from build123d import *

# Parameters (mm, degrees)
SKETCH1_W                      = 80
SKETCH1_H                      = 100
BASE_FLANGE1_DEPTH             = 3.175
EDGE_FLANGE2_STRIP_W           = 14.1732
EDGE_FLANGE2_STRIP_H           = 3.175
EDGE_FLANGE2_STRIP_CUT_DEPTH   = 80
EDGE_FLANGE2_STRIP_2_W         = 14.1732
EDGE_FLANGE2_STRIP_2_H         = 3.175
EDGE_FLANGE2_STRIP_CUT_2_DEPTH = 80
EDGE_FLANGE2_DEPTH             = 80
EDGE_FLANGE2_BEND_DEPTH        = 80
CUT_EXTRUDE1_REACH             = 155.948
SKETCH12_R                     = 28
M6_CLEARANCE_HOLE1_D           = 6.4
M6_CLEARANCE_HOLE1_DEPTH       = 3.175
M6_CLEARANCE_HOLE2_D           = 6.4
CUT_EXTRUDE2_REACH             = 155.948
SKETCH19_R                     = 11
FILLET1_R                      = 5


# Sheet-metal steps are written as plain solids
with BuildPart() as part:
    # Sketch1 → Base-Flange1 (new body)
    with BuildSketch(Plane(origin=(0, 0, 0), x_dir=(0, 0, -1), z_dir=(0, -1, 0))):
        Rectangle(SKETCH1_W, SKETCH1_H)
    extrude(amount=-BASE_FLANGE1_DEPTH)

    # Edge-Flange2 strip (across the edge) → Edge-Flange2 strip cut (cut)
    with BuildSketch(Plane(origin=(50, 3.175, 40), x_dir=(-1, 0, 0), z_dir=(0, 0, -1))):
        with Locations((-3.175, -1.5875)):
            Rectangle(EDGE_FLANGE2_STRIP_W, EDGE_FLANGE2_STRIP_H)
    extrude(amount=EDGE_FLANGE2_STRIP_CUT_DEPTH, mode=Mode.SUBTRACT)

    # Edge-Flange2 strip 2 (across the edge) → Edge-Flange2 strip cut 2 (cut)
    with BuildSketch(Plane(origin=(-50, 3.175, -40), x_dir=(1, 0, 0), z_dir=(0, 0, 1))):
        with Locations((-3.175, -1.5875)):
            Rectangle(EDGE_FLANGE2_STRIP_2_W, EDGE_FLANGE2_STRIP_2_H)
    extrude(amount=EDGE_FLANGE2_STRIP_CUT_2_DEPTH, mode=Mode.SUBTRACT)

    # Edge-Flange2 section (across the edge) → Edge-Flange2 (add)
    with BuildSketch(Plane(origin=(50, 3.175, 40), x_dir=(-1, 0, 0), z_dir=(0, 0, -1))):
        with BuildLine():
            Line((0, 0.7366), (0, 106.825))
            Line((0, 106.825), (3.175, 106.825))
            Line((3.175, 106.825), (3.175, 0.7366))
            ThreePointArc((3.175, 0.7366), (3.390745145, 0.215745145), (3.9116, 0))
            Line((3.9116, 0), (3.9116, -3.175))
            ThreePointArc((3.9116, -3.175), (1.145681115, -2.029318885), (0, 0.7366))
        make_face()
    extrude(amount=EDGE_FLANGE2_DEPTH)

    # Edge-Flange2 section 2 (across the edge) → Edge-Flange2 bend (add)
    with BuildSketch(Plane(origin=(-50, 3.175, -40), x_dir=(1, 0, 0), z_dir=(0, 0, 1))):
        with BuildLine():
            Line((0, 0.7366), (0, 106.825))
            Line((0, 106.825), (3.175, 106.825))
            Line((3.175, 106.825), (3.175, 0.7366))
            ThreePointArc((3.175, 0.7366), (3.390745145, 0.215745145), (3.9116, 0))
            Line((3.9116, 0), (3.9116, -3.175))
            ThreePointArc((3.9116, -3.175), (1.145681115, -2.029318885), (0, 0.7366))
        make_face()
    extrude(amount=EDGE_FLANGE2_BEND_DEPTH)

    # Sketch12 → Cut-Extrude1 (cut, up to next)
    with BuildSketch(Plane(origin=(50, 0, 0), x_dir=(0, 0, -1), z_dir=(1, 0, 0)), mode=Mode.PRIVATE) as cut_extrude1_sk1:
        with BuildLine():
            Line((-40, 110), (-40, 70))
            ThreePointArc((-40, 70), (-28.284271269, 98.284271226), (-6.1e-08, 110))
            Line((-6.1e-08, 110), (-40, 110))
        make_face()
    cut_extrude1_tool1 = extrude(cut_extrude1_sk1.sketch, amount=-CUT_EXTRUDE1_REACH, mode=Mode.PRIVATE) & part.part
    # Sketch12 → Cut-Extrude1 (cut, up to next)
    with BuildSketch(Plane(origin=(50, 0, 0), x_dir=(0, 0, -1), z_dir=(1, 0, 0)), mode=Mode.PRIVATE) as cut_extrude1_sk2:
        with BuildLine():
            Line((40, 110), (-6.1e-08, 110))
            ThreePointArc((-6.1e-08, 110), (28.284271226, 98.284271269), (40, 70))
            Line((40, 70), (40, 110))
        make_face()
    cut_extrude1_tool2 = extrude(cut_extrude1_sk2.sketch, amount=-CUT_EXTRUDE1_REACH, mode=Mode.PRIVATE) & part.part
    # Sketch12 → Cut-Extrude1 (cut, up to next)
    with BuildSketch(Plane(origin=(50, 0, 0), x_dir=(0, 0, -1), z_dir=(1, 0, 0)), mode=Mode.PRIVATE) as cut_extrude1_sk3:
        with Locations(Location((0, 70, 0), (0, 0, 90))):
            Circle(SKETCH12_R)
    cut_extrude1_tool3 = extrude(cut_extrude1_sk3.sketch, amount=-CUT_EXTRUDE1_REACH, mode=Mode.PRIVATE) & part.part
    add(cut_extrude1_tool1.solids().sort_by_distance((50, 101.065282, 31.065282))[0], mode=Mode.SUBTRACT)
    add(cut_extrude1_tool2.solids().sort_by_distance((50, 101.065282, -31.065282))[0], mode=Mode.SUBTRACT)
    add(cut_extrude1_tool3.solids().sort_by_distance((50, 70, 0))[0], mode=Mode.SUBTRACT)

    # M6 Clearance Hole1
    with Locations(Plane(origin=(50, 70, 32.5), x_dir=(0, 1, 0), z_dir=(1, 0, 0))):
        with Locations((0, 0), (-32.5, -32.5), (0, -65), (32.5, -32.5)):
            Hole(M6_CLEARANCE_HOLE1_D / 2, depth=M6_CLEARANCE_HOLE1_DEPTH)

    # M6 Clearance Hole2 (through all)
    with Locations(Plane(origin=(-35, 0, 30), x_dir=(0, 0, -1), z_dir=(0, -1, 0))):
        with Locations((0, 0), (0, 70), (60, 0), (60, 70)):
            Hole(M6_CLEARANCE_HOLE2_D / 2)

    # Sketch19 → Cut-Extrude2 (cut, up to next)
    with BuildSketch(Plane.ZY.offset(50), mode=Mode.PRIVATE) as cut_extrude2_sk1:
        with BuildLine():
            Line((-40, 40), (-17.398181668, 79.864242224))
            ThreePointArc((-17.398181668, 79.864242224), (0, 90), (17.398181668, 79.864242224))
            Line((17.398181668, 79.864242224), (40, 40))
            Line((40, 40), (40, 110))
            Line((40, 110), (-40, 110))
            Line((-40, 110), (-40, 40))
        make_face()
    cut_extrude2_tool1 = extrude(cut_extrude2_sk1.sketch, amount=-CUT_EXTRUDE2_REACH, mode=Mode.PRIVATE) & part.part
    # Sketch19 → Cut-Extrude2 (cut, up to next)
    with BuildSketch(Plane.ZY.offset(50), mode=Mode.PRIVATE) as cut_extrude2_sk2:
        with Locations(Location((0, 70, 0), (0, 0, 270))):
            Circle(SKETCH19_R)
    cut_extrude2_tool2 = extrude(cut_extrude2_sk2.sketch, amount=-CUT_EXTRUDE2_REACH, mode=Mode.PRIVATE) & part.part
    # Sketch19 → Cut-Extrude2 (cut, up to next)
    with BuildSketch(Plane.ZY.offset(50), mode=Mode.PRIVATE) as cut_extrude2_sk3:
        with BuildLine():
            ThreePointArc((-11.390381057, 62), (-12.990381057, 60.4), (-14.590381057, 62))
            Line((-14.590381057, 62), (-14.590381057, 63))
            ThreePointArc((-14.590381057, 63), (-12.990381057, 64.6), (-11.390381057, 63))
            Line((-11.390381057, 63), (-11.390381057, 62))
        make_face()
    cut_extrude2_tool3 = extrude(cut_extrude2_sk3.sketch, amount=-CUT_EXTRUDE2_REACH, mode=Mode.PRIVATE) & part.part
    # Sketch19 → Cut-Extrude2 (cut, up to next)
    with BuildSketch(Plane.ZY.offset(50), mode=Mode.PRIVATE) as cut_extrude2_sk4:
        with BuildLine():
            ThreePointArc((14.590381057, 62), (12.990381057, 60.4), (11.390381057, 62))
            Line((11.390381057, 62), (11.390381057, 63))
            ThreePointArc((11.390381057, 63), (12.990381057, 64.6), (14.590381057, 63))
            Line((14.590381057, 63), (14.590381057, 62))
        make_face()
    cut_extrude2_tool4 = extrude(cut_extrude2_sk4.sketch, amount=-CUT_EXTRUDE2_REACH, mode=Mode.PRIVATE) & part.part
    # Sketch19 → Cut-Extrude2 (cut, up to next)
    with BuildSketch(Plane.ZY.offset(50), mode=Mode.PRIVATE) as cut_extrude2_sk5:
        with BuildLine():
            ThreePointArc((1.6, 84.5), (0, 82.9), (-1.6, 84.5))
            Line((-1.6, 84.5), (-1.6, 85.5))
            ThreePointArc((-1.6, 85.5), (0, 87.1), (1.6, 85.5))
            Line((1.6, 85.5), (1.6, 84.5))
        make_face()
    cut_extrude2_tool5 = extrude(cut_extrude2_sk5.sketch, amount=-CUT_EXTRUDE2_REACH, mode=Mode.PRIVATE) & part.part
    add(cut_extrude2_tool1.solids().sort_by_distance((-50, 60.456413, -29.623817))[0], mode=Mode.SUBTRACT)
    add(cut_extrude2_tool2.solids().sort_by_distance((-50, 70, 0))[0], mode=Mode.SUBTRACT)
    add(cut_extrude2_tool3.solids().sort_by_distance((-50, 62.5, -12.990381))[0], mode=Mode.SUBTRACT)
    add(cut_extrude2_tool4.solids().sort_by_distance((-50, 62.5, 12.990381))[0], mode=Mode.SUBTRACT)
    add(cut_extrude2_tool5.solids().sort_by_distance((-50, 85, 0))[0], mode=Mode.SUBTRACT)

    # Fillet1
    fillet1_edges = [part.edges().sort_by_distance(p)[0] for p in [
        (-48.4125, 40, 40),
        (-48.4125, 40, -40),
    ]]
    fillet(fillet1_edges, radius=FILLET1_R)


solid = part.part
Part model, mm, in its own coordinate system. A direction names the side the tool comes from. Coordinates: 2 decimals unless noted, no trailing zeros. Loops run counter-clockwise (first coordinate to the right, second up) from the corner with the lowest first, then second, coordinate; pieces in that order, holes last. Notation, with made-up numbers: (12, 2) -> (22, 2) arc R28 cw to (22, 41) -> close; hole circle Ø10 at (88.5, 9). An arc over 180 degrees is marked (long way). Use a Markdown table: item, result. Add a question column.
Item 1: Which spindle directions (+Z, -Z, +X, -X, +Y, -Y) get a long thin tool onto all of the face, cutting with end or side? Do faces 4 (the cylindrical face through (-48.4, 82.9, 0)), 5 (the flat face through (1, 3.175, 1)), 6 (the cylindrical face through (48, 40, 2)), 7 (the flat face through (-48.43, 60.78, 28.22)), 8 (the flat face through (-48.43, 60.23, -28.53)). Say none if no direction does.
Item 2: Band-saw the part on A-A on x = 35. Write the cut outline in (y, z) (3 decimals).
Item 3: Band-saw the part on B-B on y = 13. Write the cut outline in (x, z) (3 decimals).
Item 4: Band-saw the part on D-D on z = 31. Write the cut outline in (x, y) (3 decimals), plus the area to 3 significant figures.
Item 5: Probe probe 1 along Z at (x, y) = (48, 70); probe 2 along X at (y, z) = (31.5, 0.5) (3 decimals); probe 3 along X at (y, z) = (2.2, 30). List the from-to ranges inside material, lowest first.
Item 6: Pull direction X, two halves, no side cores. Call faces 1 (the cylindrical face through (-48.4, 64.6, -13)), 2 (the flat face through (-46.825, 38, -1)), 3 (the flat face through (-50, 37, -1)): +X half, -X half, draft (parallel to the pull), parting line (faces both ways), or undercut.
Item 7: Flat gauge pins, fed straight in: P1, Ø4, axis at y = 102.5, z = 0, coming from the +X side; P2, Ø0.8, axis at x = -48, y = 62.5, coming from the -Z side; P3, Ø1.1, axis at x = -47.5, y = 62.5, coming from the +Z side (3 decimals); P4, Ø0.8, axis at x = -48, y = 62.5, coming from the +Z side. Where does each tip first touch, or does it go through?
Item 8: Band-saw the part on C-C on y = 49.5. Write the cut outline in (x, z) (3 decimals).
Geometry says:
| question | item | result |
|---|---|---|
| 1 | face 4 | +X, -X |
| 1 | face 5 | +Z, -Z, +Y |
| 1 | face 6 | +X |
| 1 | face 7 | +Z, -X, +Y |
| 1 | face 8 | -Z, -X, +Y |
| 2 | outline | (0, -40) -> (3.175, -40) -> (3.175, -33.2) -> (0, -33.2) -> close; (0, -26.8) -> (3.175, -26.8) -> (3.175, 26.8) -> (0, 26.8) -> close; (0, 33.2) -> (3.175, 33.2) -> (3.175, 40) -> (0, 40) -> close |
| 3 | outline | (-50, -40) -> (-46.825, -40) -> (-46.825, 40) -> (-50, 40) -> close; (46.825, -40) -> (50, -40) -> (50, 40) -> (46.825, 40) -> close |
| 4 | outline | (-50, 3.912) arc R3.912 ccw to (-46.088, 0) -> (-38.04, 0) -> (-38.04, 3.175) -> (-46.088, 3.175) arc R0.737 cw to (-46.825, 3.912) -> (-46.825, 55.874) -> (-50, 55.874) -> close; (-31.96, 0) -> (31.96, 0) -> (31.96, 3.175) -> (-31.96, 3.175) -> close; (38.04, 0) -> (46.088, 0) arc R3.912 ccw to (50, 3.912) -> (50, 67.173) -> (46.825, 67.173) -> (46.825, 3.912) arc R0.737 cw to (46.088, 3.175) -> (38.04, 3.175) -> close; (46.825, 72.827) -> (50, 72.827) -> (50, 95.278) -> (46.825, 95.278) -> close |
| 4 | area | 714 mm² |
| 5 | probe 1 | -40 to -35.7, -29.3 to -28, 28 to 29.3, 35.7 to 40 |
| 5 | probe 2 | -50 to -46.825, 46.825 to 50 |
| 5 | probe 3 | -49.61 to -38.2, -31.8 to 31.8, 38.2 to 49.61 |
| 6 | face 1 | draft |
| 6 | face 2 | undercut |
| 6 | face 3 | -X half |
| 7 | P1 | through |
| 7 | P2 | z = -27.47 |
| 7 | P3 | z = 27.555 |
| 7 | P4 | z = 27.47 |
| 8 | outline | (-50, -34.614) -> (-46.825, -34.614) -> (-46.825, 34.614) -> (-50, 34.614) -> close; (46.825, -40) -> (50, -40) -> (50, -19.072) -> (46.825, -19.072) -> close; (46.825, 19.072) -> (50, 19.072) -> (50, 40) -> (46.825, 40) -> close |
